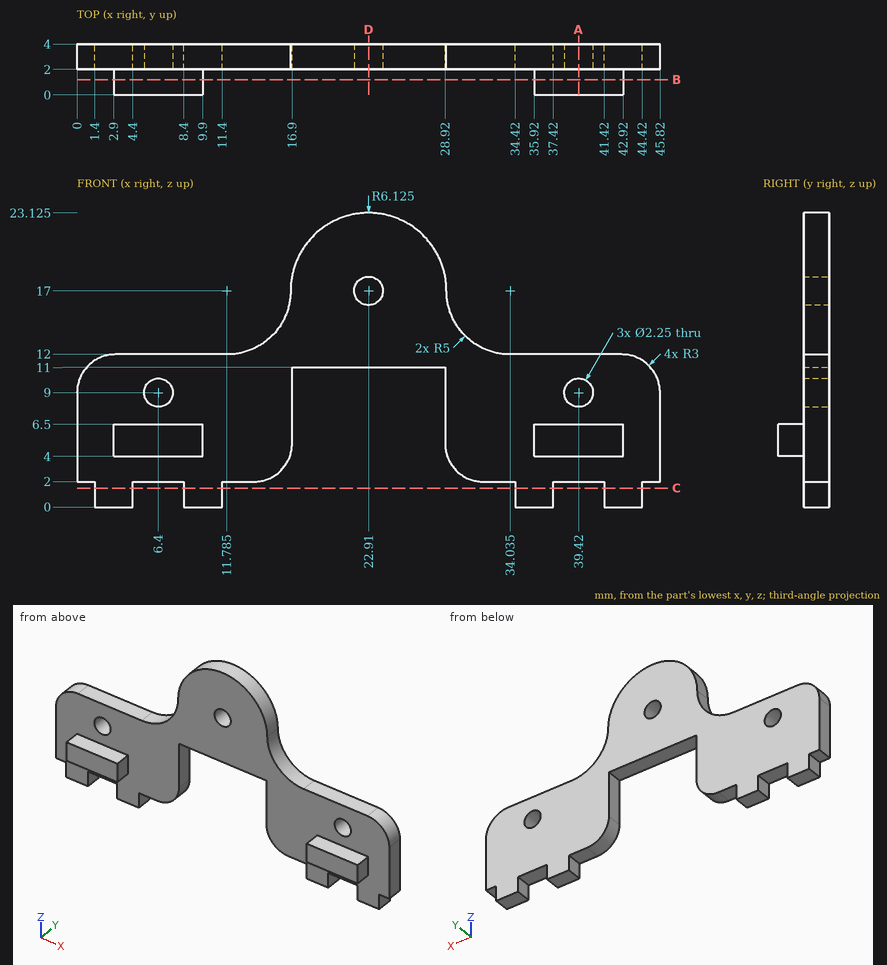
Study the drawing (mm; zero at the part's minimum x, y, z) and answer. Give positions to 0.01 mm unless a question says otherwise; leave off trailing zeros. Loops run counter-clockwise (first coordinate to the right, second up) from the corner with the lowest first, then second, coordinate; pieces in that order, holes last. Notation, with made-up numbers: M 61,73.25 L 93,73.25 A18 cw 93,89.25 Z; hole C 12.25,73 d5. An arc over 180 degrees is marked long. Use CSV: the item, a comma, the result in double quotes.
1) Find section D-D on x = 22.91. Write down the section's boundary in (y, z) (3 decimals).
Answer:
outline,"M 2,11 L 4,11 L 4,15.875 L 2,15.875 Z; M 2,18.125 L 4,18.125 L 4,23.125 L 2,23.125 Z"
2) Find section A-A on x = 39.42. Write down the section's boundary in (y, z) (3 decimals).
Answer:
outline,"M 0,4 L 2,4 L 2,2 L 4,2 L 4,7.875 L 2,7.875 L 2,6.5 L 0,6.5 Z; M 2,10.125 L 4,10.125 L 4,12 L 2,12 Z"
3) Find section B-B on y = 1.2. Write down the section's boundary in (x, z).
Answer:
outline,"M 2.9,4 L 9.9,4 L 9.9,6.5 L 2.9,6.5 Z; M 35.92,4 L 42.92,4 L 42.92,6.5 L 35.92,6.5 Z"
4) Find section C-C on z = 1.5. Write down the section's boundary in (x, y).
Answer:
outline,"M 1.4,2 L 4.4,2 L 4.4,4 L 1.4,4 Z; M 8.4,2 L 11.4,2 L 11.4,4 L 8.4,4 Z; M 34.42,2 L 37.42,2 L 37.42,4 L 34.42,4 Z; M 41.42,2 L 44.42,2 L 44.42,4 L 41.42,4 Z"
5) Consider L1, parallel to X at y = 3.5, z = 9 (3 decimals); L2, parallel to Z at x = 39.42, y = 2.4 (3 decimals); L3, parallel to X at y = 2.5, z = 17 (3 decimals). Determine where each line is inside the solid, lowest interval first.
Answer:
L1,"0 to 5.275, 7.525 to 16.9, 28.92 to 38.295, 40.545 to 45.82"
L2,"2 to 7.875, 10.125 to 12"
L3,"16.785 to 21.785, 24.035 to 29.035"
6) Given P1, Ø2, axis at x = 14, z = 14.5, coming from the -Y side; P2, Ø2, axis at x = 24, y = 3, coming from the -Z side; P3, Ø2, axis at y = 3, z = 0.5, coming from the +X side; P4, Ø2, axis at y = 0.5, z = 6, coming from the +X side, each flat-ended and moving along its own axis, determine where each tip first touches the part or whether it passes through.
Answer:
P1,"through"
P2,"z = 11"
P3,"x = 44.42"
P4,"x = 42.92"
